from build123d import *
from build123d.topology import SkipClean

# Parameters (mm, degrees)
SKETCH1_R           = 31.75
BOSS_EXTRUDE1_DEPTH = 38.1
CUT_EXTRUDE1_DEPTH  = 59.887477446
FILLET1_R           = 12.7
SKETCH7_R           = 5.5626
CUT_EXTRUDE2_DEPTH  = 75.053089233
SKETCH8_R           = 4.445
BOSS_EXTRUDE2_DEPTH = 3.175


with BuildPart() as part:
    # Sketch1 → Boss-Extrude1 (new body)
    with BuildSketch(Plane(origin=(0, 0, 0), x_dir=(1, 0, 0), z_dir=(0, 1, 0))):
        with Locations(Location((0, 0, 0), (0, 0, 90))):
            Circle(SKETCH1_R)
    extrude(amount=BOSS_EXTRUDE1_DEPTH)

    # Sketch2 → Cut-Extrude1 (cut, through all)
    with BuildSketch(Plane.XZ):
        with BuildLine():
            Line((-15.875, 27.49630657), (15.875, 27.49630657))
            ThreePointArc((15.875, 27.49630657), (0, 31.75), (-15.875, 27.49630657))
        make_face()
        with BuildLine():
            Line((-15.875, -27.49630657), (15.875, -27.49630657))
            ThreePointArc((15.875, -27.49630657), (0, -31.75), (-15.875, -27.49630657))
        make_face()
    extrude(amount=-CUT_EXTRUDE1_DEPTH, mode=Mode.SUBTRACT)

    # Fillet1
    fillet1_edges = [part.edges().sort_by_distance(p)[0] for p in [
        (-31.75, 38.1, 0),
        (0, 38.1, -27.49630657),
        (31.75, 38.1, 0),
        (0, 38.1, 27.49630657),
    ]]
    fillet(fillet1_edges, radius=FILLET1_R)

    # Sketch4 → 1/4 NPT Tapped Hole1 (revolve, cut)
    with BuildSketch(Plane(origin=(0, 12.7, 27.49630657), x_dir=(0, -1, 0), z_dir=(1, 0, 0))):
        Polygon((0, 0), (0, 20.360347279), (5.5626, 17.018), (5.5626, 9.906), (6.557984794, 9.906), (6.8545837, 0), align=None)
    f_1_4_npt_tapped_hole1 = revolve(axis=Axis((0, 12.7, 33.84630657), (0, 0, -1)), mode=Mode.SUBTRACT)

    # Mirror1: 1/4 NPT Tapped Hole1 across plane
    add(f_1_4_npt_tapped_hole1.mirror(Plane.XY), mode=Mode.SUBTRACT)

    # Sketch6 → 1/4 NPT Tapped Hole2 (revolve, cut)
    with BuildSketch(Plane(origin=(-26.85868109, 12.7, 16.931442647), x_dir=(0.5332737841578493, 0, 0.8459427114940868), z_dir=(0, 1, 0))):
        Polygon((0, 0), (0, 20.360347279), (5.5626, 17.018), (5.5626, 9.906), (6.557984794, 9.906), (6.8545837, 0), align=None)
    revolve(axis=Axis((-32.230417308, 12.7, 20.317731176), (0.8459427114940866, 0, -0.5332737841578492)), mode=Mode.SUBTRACT)

    # Sketch6 at point 2 (carried to point 2, square into its face) → 1/4 NPT Tapped Hole2 at 2 (revolve, cut)
    with BuildSketch(Plane(origin=(-26.85868109, 12.7, -16.931442647), x_dir=(-0.533273808, 0, 0.845942696), z_dir=(0, 1, 0))):
        Polygon((0, 0), (0, 20.360347279), (5.5626, 17.018), (5.5626, 9.906), (6.557984794, 9.906), (6.8545837, 0), align=None)
    revolve(axis=Axis((-32.230417211, 12.7, -20.317731331), (0.845942696, 0, 0.533273808)), mode=Mode.SUBTRACT)

    # Sketch7 → Cut-Extrude2 (cut, through all)
    with SkipClean():  # the faces are left unmerged after this step: merging them gives an invalid solid
        with BuildSketch(Plane(origin=(0, 0, -27.49630657), x_dir=(-1, 0, 0), z_dir=(0, 0, -1))):
            with Locations(Location((0, 12.7, 0), (0, 0, 180))):
                Circle(SKETCH7_R)
        extrude(amount=-CUT_EXTRUDE2_DEPTH, mode=Mode.SUBTRACT)

    # Sketch8 → Boss-Extrude2 (add)
    with SkipClean():  # the faces are left unmerged after this step: merging them gives an invalid solid
        with BuildSketch(Plane(origin=(0, 38.1, 0), x_dir=(1, 0, 0), z_dir=(0, 1, 0))):
            with Locations(Location((0, 0, 0), (0, 0, 270))):
                Circle(SKETCH8_R)
        extrude(amount=BOSS_EXTRUDE2_DEPTH)


solid = part.part
Here's how the part is built. I have some questions about the finished solid (model axes, mm). A direction names the side the tool comes from. Coordinates: 2 decimals unless noted, no trailing zeros. Write each loop counter-clockwise with the first axis right and the second up, starting at its lowest first coordinate (ties: lowest second). Pieces come first, ordered by that corner, then holes.
1) If I drill on line 1 (Y direction, x = 0, z = 12); line 2 (Y direction, x = 0, z = -2.5) (3 decimals); line 3 (Z direction, x = 4.5, y = 8), over which ranges is the centre line in solid material (lowest first)?
Filled in:
line 1: y = 0 to 7.14, 18.26 to 38.1
line 2: y = 0 to 7.137, 18.263 to 41.275
line 3: z = -17.59 to 17.59
2) Thinking about a two-plate mould opening in X: for faces 1 (the face through (31.747, 12.522, 0.465)), 2 (the face through (0, 41.275, 0)), 3 (the face through (-0.3, 19.4, 22.6)), which applies, +X half, -X half, draft (parallel to the pull), parting line (faces both ways), or undercut?
Filled in:
face 1: +X half
face 2: draft
face 3: undercut
3) If we section it at B-B (x = 8.5): List the corners of the cut face in (y, z) for me, plus the area to 3 significant figures.
Filled in:
outline: (0, -27.5) - (25.4, -27.5) arc R12.7 ccw to (38.1, -14.8) - (38.1, 14.8) arc R12.7 ccw to (25.4, 27.5) - (0, 27.5) - close
area: 2,030 mm2
4) If we section it at C-C (y = 21.5): List the corners of the cut face in (x, z) for me (3 decimals), plus the area to 3 significant figures.
Filled in:
outline: (-15.875, -27.496) - (15.875, -27.496) arc R31.75 ccw to (15.875, 27.496) - (-15.875, 27.496) arc R31.75 ccw to start
area: 2,980 mm2
5) Which directions (+Z, -Z, +X, -X, +Y, -Y) give clear straight access to the entire face, cutting with the end or side of a thin tool? Please do faces 4 (the face through (-9.9, 13.6, 6.8)), 5 (the face through (-4.34, 39.67, -0.96)), 6 (the face through (5, 16, -17.59)).
Filled in:
face 4: none
face 5: +Y
face 6: -Z
6) If we section it at D-D (z = -8): Count the separate pieces of the cut face and the enclosed holes in it, plus the area to 3 significant figures.
Filled in:
separate pieces: 1
enclosed holes: 2
area: 2,040 mm2
7) If we section it at A-A (z = 0): List the corners of the cut face in (x, y) for me (3 decimals), plus the area to 3 significant figures.
Filled in:
outline: (-31.75, 0) - (31.75, 0) - (31.75, 25.4) arc R12.7 ccw to (19.05, 38.1) - (4.445, 38.1) - (4.445, 41.275) - (-4.445, 41.275) - (-4.445, 38.1) - (-19.05, 38.1) arc R12.7 ccw to (-31.75, 25.4) - close; hole circle Ø11.125 at (0, 12.7)
area: 2,280 mm2
8) I'm going to push flat-ended pins straight in: pin 1 (1 mm diameter, centred on y = 20, z = 18, fed in from +X); pin 2 (6.5 mm diameter, centred on x = 0, y = 12.7, fed in from +Z); pin 3 (3 mm diameter, centred on y = 33.5, z = -4, fed in from -X); pin 4 (1.5 mm diameter, centred on y = 17.5, z = 6, fed in from -X). Where does each tip first touch, or does it pass through?
Filled in:
pin 1: stops at x = 26.49
pin 2: passes through
pin 3: stops at x = -29.65
pin 4: stops at x = -31.31
